Check sheet for the modelled part. Datum: model origin and axes. Units: mm. Round coordinates to 2 decimals unless told otherwise and drop trailing zeros. Write each loop counter-clockwise with the first axis right and the second up, starting at its lowest first coordinate (ties: lowest second). Pieces come first, ordered by that corner, then holes.
Item 1: Release check for a two-part mould opening along Z. For faces 1 (the cylindrical face through (-29.9, 0, 9.6)), 2 (the flat face through (22.5, 0, 0)), 3 (the cylindrical face through (-29.9, -0.02, 11.75)), 4 (the cylindrical face through (0.29, 0.1, -13.75)) record: +Z half, -Z half, draft (parallel to the pull), parting line (faces both ways), or undercut.
Item 2: Material ranges on line 1 (X direction, y = -2.25, z = -0.25); line 2 (Z direction, x = -15.5, y = 3.25); line 3 (X direction, y = -3.75, z = 3), recorded low to high.
Item 3: Cross-section at A-A on z = -3.75. Enter the section's corners in (x, y), plus the area to 3 significant figures.
Item 4: Cross-section at C-C on x = -28. Enter the section's corners in (y, z) (3 decimals).
Item 5: Go/stop test with flat-tipped pins: pin 1 Ø1.5 at (x, y) = (-11.5, 1) entering from -Z; pin 2 Ø3 at (y, z) = (0, -3) entering from -X; pin 3 Ø1.5 at (x, y) = (16, -2) entering from +Z. Record where each tip stops, or that it passes through.
Item 6: Cross-section at B-B on x = 13. Enter the section's corners in (y, z), plus the area to 3 significant figures.
from build123d import *

# Parameters (mm, degrees)
BOSS_EXTRUDE1_DEPTH = 22.5
FILLET1_R           = 2
BOSS_EXTRUDE2_DEPTH = 15


with BuildPart() as part:
    # Sketch1 → Boss-Extrude1 (new, symmetric)
    with BuildSketch(Plane(origin=(0, 0, 0), x_dir=(0, 0, -1), z_dir=(1, 0, 0))):
        with BuildLine():
            Line((-9, 4.75), (9, 4.75))
            ThreePointArc((9, 4.75), (13.75, 0), (9, -4.75))
            Line((9, -4.75), (-9, -4.75))
            ThreePointArc((-9, -4.75), (-13.75, 0), (-9, 4.75))
        make_face()
    extrude(amount=BOSS_EXTRUDE1_DEPTH, both=True)

    # Fillet1
    fillet1_edges = [part.edges().sort_by_distance(p)[0] for p in [
        (22.5, 0, -13.75),
        (22.5, 4.75, 0),
        (22.5, 0, 13.75),
        (-22.5, 4.75, 0),
        (-22.5, 0, -13.75),
        (-22.5, -4.75, 0),
        (-22.5, 0, 13.75),
        (22.5, -4.75, 0),
    ]]
    fillet(fillet1_edges, radius=FILLET1_R)

    # Sketch2 → Boss-Extrude2 (add)
    with BuildSketch(Plane.ZY.offset(22.5)):
        with BuildLine():
            ThreePointArc((10.675, 0.283945417), (9.6, 0), (10.675, -0.283945417))
            ThreePointArc((10.675, -0.283945417), (11.75, 0), (10.675, 0.283945417))
        make_face()
    extrude(amount=BOSS_EXTRUDE2_DEPTH)


solid = part.part
Response values:
1. face 1: undercut
1. face 2: draft
1. face 3: undercut
1. face 4: -Z half
2. line 1: x = -22.5 to 22.5
2. line 2: z = -12.46 to 12.46
2. line 3: x = -22.23 to 22.23
3. outline: (-22.5, -2.75) arc R2 ccw to (-20.5, -4.75) - (20.5, -4.75) arc R2 ccw to (22.5, -2.75) - (22.5, 2.75) arc R2 ccw to (20.5, 4.75) - (-20.5, 4.75) arc R2 ccw to (-22.5, 2.75) - close
3. area: 424 mm2
4. outline: (-0.284, 10.675) arc R0.575 ccw (long way) to (0.284, 10.675) arc R0.575 ccw (long way) to start
5. pin 1: stops at z = -13.74
5. pin 2: stops at x = -22.5
5. pin 3: stops at z = 13.58
6. outline: (-4.75, -9) arc R4.75 ccw to (4.75, -9) - (4.75, 9) arc R4.75 ccw to (-4.75, 9) - close
6. area: 242 mm2
